Here's the drawing with two shaded views (mm, measured from the low corner). I have some questions. Give positions to 0.01 mm unless a question says otherwise; leave off trailing zeros. Write each loop counter-clockwise with the first axis right and the second up, starting at its lowest first coordinate (ties: lowest second). Pieces come first, ordered by that corner, then holes. Notation, with made-up numbers: (48, 36) -> (73, 36) arc R13 cw to (73, 61) -> close; hole circle Ø1 at (4, 67). An arc over 180 degrees is marked (long way). Put each result on its own line as item: value. Start each with the question number.
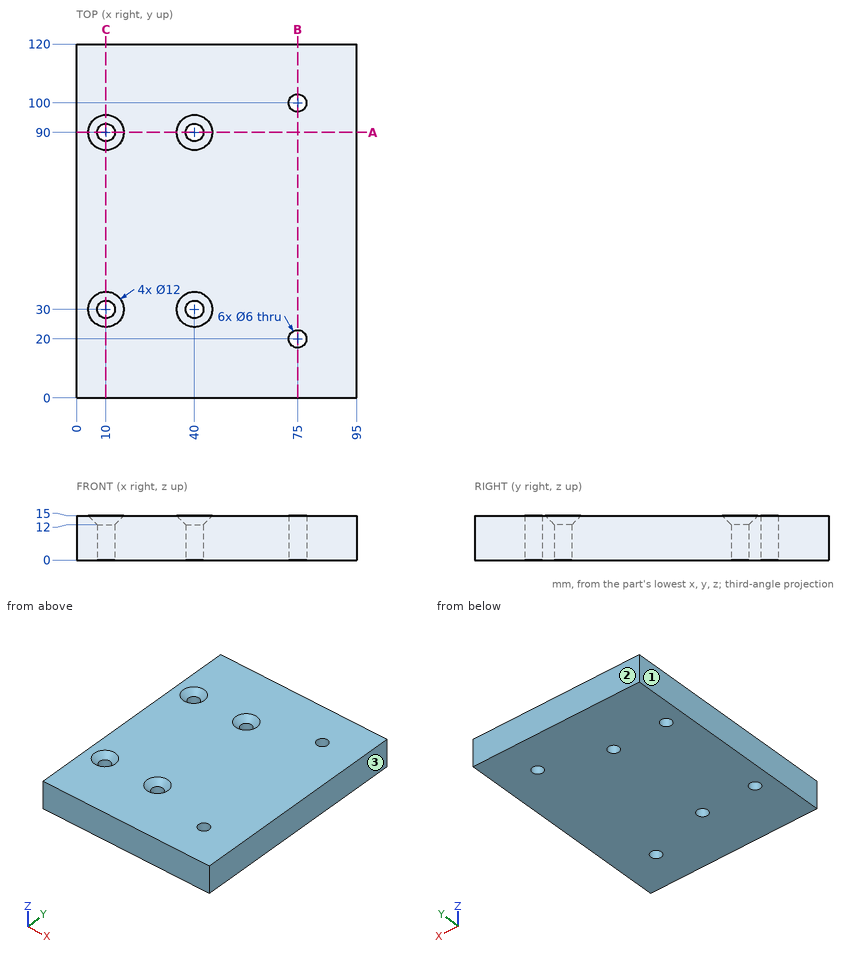
1) I'm going to push a flat-ended pin straight in: pin 1 Ø5 at (x, y) = (40, 30) entering from -Z. Where does the tip first touch, or does it pass through?
2) Thinking about a two-plate mould opening in X: for the marked faces 1, 2 and 3, which applies, released by +X, released by -X, zero draft, split by the parting line, or undercut?
3) I want a section at C-C, the plane x = 10. Write out the boundary of the cut face in (y, z).
4) I want a section at A-A, the plane y = 90. Write out the boundary of the cut face in (x, z), and give its area (3 significant figures).
5) I want a section at B-B, the plane x = 75. Write out the boundary of the cut face in (y, z), and give its area (3 significant figures).
6) I need wall thicknesses on probe 1 along X at (y, z) = (30, 4.5); probe 2 along Y at (x, z) = (75, 7.25); probe 3 along Y at (x, z) = (40, 3.75). Which ranges of each line are inside material? Lowest first, please.
Established:
1. pin 1: passes through
2. face 1: released by -X
2. face 2: zero draft
2. face 3: released by +X
3. outline: (0, 0) -> (27, 0) -> (27, 12) -> (24, 15) -> (0, 15) -> close; (33, 0) -> (87, 0) -> (87, 12) -> (84, 15) -> (36, 15) -> (33, 12) -> close; (93, 0) -> (120, 0) -> (120, 15) -> (96, 15) -> (93, 12) -> close
4. outline: (0, 0) -> (7, 0) -> (7, 12) -> (4, 15) -> (0, 15) -> close; (13, 0) -> (37, 0) -> (37, 12) -> (34, 15) -> (16, 15) -> (13, 12) -> close; (43, 0) -> (95, 0) -> (95, 15) -> (46, 15) -> (43, 12) -> close
4. area: 1,230 mm2
5. outline: (0, 0) -> (17, 0) -> (17, 15) -> (0, 15) -> close; (23, 0) -> (97, 0) -> (97, 15) -> (23, 15) -> close; (103, 0) -> (120, 0) -> (120, 15) -> (103, 15) -> close
5. area: 1,620 mm2
6. probe 1: x = 0 to 7, 13 to 37, 43 to 95
6. probe 2: y = 0 to 17, 23 to 97, 103 to 120
6. probe 3: y = 0 to 27, 33 to 87, 93 to 120
